Geometry check sheet. Reference: the model listing, model coordinates, mm. A direction names the side the tool comes from. Round coordinates to 2 decimals unless told otherwise and drop trailing zeros. Write each loop counter-clockwise with the first axis right and the second up, starting at its lowest first coordinate (ties: lowest second). Pieces come first, ordered by that corner, then holes. Notation, with made-up numbers: M 40.5,57.5 L 94.5,57.5 A26 ccw 94.5,92.5 Z; hole C 1,-25 d10. An arc over 180 degrees is marked long. Put each result on its own line as item: value. Start each with the question number.
(1) Section check D-D on x = 3.5. Record the cut outline in (y, z), then the cut area to 3 significant figures.
(2) Tool access check on faces 4 (the flat face through (-19.404, -19.269, 5.358)), 5 (the flat face through (9.525, 27, 5)), 6 (the flat face through (2, 31, 2.54)), 7 (the flat face through (0, 0, 2.54)), 8 (the flat face through (8.273, 28.333, 7.862)). Record the directions out of +Z, -Z, +X, -X, +Y, -Y that give a thin tool (end or side, any length) a straight path to the whole face; none if there is none.
(3) Mould release check, pull along Y, two halves, no side actions. Record for faces 1 (the flat face through (-28, -14, 2.54)), 2 (the flat face through (-9.525, 27, 5)), 3 (the flat face through (28.674, -7.002, 7.862)): pulls with the +Y half, pulls with the -Y half, needs draft (parallel to the pull), parting line crosses it, or undercut.
(4) Section check A-A on z = 26. Record the cut outline in (x, y) (1 decimal), then the cut area to 3 significant figures.
(5) Material ranges on probe 1 along X at (y, z) = (25.5, 10) (3 decimals); probe 2 along X at (y, z) = (-6, 11); probe 3 along Y at (x, z) = (0, 1.35), recorded low to high.
(6) Section check B-B on y = 0. Record the cut outline in (x, z) (3 decimals), then the cut area to 3 significant figures.
(7) Gauge pin test, flat ends, axial feed: pin 1 (3 mm diameter, centred on x = -5.5, z = 9, fed in from -Y); pin 2 (1 mm diameter, centred on y = 17.5, z = 18, fed in from -X); pin 3 (5 mm diameter, centred on y = 28, z = 9.5, fed in from +X) (3 decimals). Record the tip position at first contact, or that the pin passes through.
(8) Section check C-C on x = 18. Record the cut outline in (y, z) (3 decimals).
from build123d import *

# Parameters (mm, degrees)
F0_R     = 21.082
F0_R_2   = 2.38125
F1_DEPTH = 2.54
F2_DEPTH = 33.02
F4_DEPTH = 2.54
F6_COUNT = 3
F6_ANGLE = 240


with BuildPart() as f1:
    # F0 (on Top) → F1 (new body)
    with BuildSketch(Plane.XY):
        with BuildLine():
            Line((-9.525, 22.86), (9.525, 22.86))
            ThreePointArc((9.525, 22.86), (0, 24.765), (-9.525, 22.86))
        make_face()
        with BuildLine():
            ThreePointArc((20.6097123392, 13.7311682786), (15.7435419805, 19.1166448654), (9.525, 22.86))
            Line((9.525, 22.86), (-9.525, 22.86))
            ThreePointArc((-9.525, 22.86), (-15.7435419805, 19.1166448654), (-20.6097123392, 13.7311682786))
            ThreePointArc((-20.6097123392, 13.7311682786), (-20.059758407, 13.154112914), (-19.8596191247, 12.3825))
            ThreePointArc((-19.8596191247, 12.3825), (-20.631435956, 11.0205832558), (-22.1963967225, 10.9829503112))
            ThreePointArc((-22.1963967225, 10.9829503112), (-24.4272710788, 4.075984868), (-24.5598407305, -3.181108029))
            Line((-24.5598407305, -3.181108029), (-15.0348407305, -19.678891971))
            ThreePointArc((-15.0348407305, -19.678891971), (-8.6837290983, -23.1926297333), (-1.5866843833, -24.7141185897))
            ThreePointArc((-1.5866843833, -24.7141185897), (0, -23.1775), (1.5866843833, -24.7141185897))
            ThreePointArc((1.5866843833, -24.7141185897), (8.6837290983, -23.1926297333), (15.0348407305, -19.678891971))
            Line((15.0348407305, -19.678891971), (24.5598407305, -3.181108029))
            ThreePointArc((24.5598407305, -3.181108029), (24.7136569602, -1.5938584173), (24.765, 0))
            ThreePointArc((24.765, 0), (24.1143006309, 5.6396569119), (22.1963967225, 10.9829503112))
            ThreePointArc((22.1963967225, 10.9829503112), (20.0723037962, 11.58875), (20.6097123392, 13.7311682786))
        make_face()
        Circle(F0_R, mode=Mode.SUBTRACT)
        with BuildLine():
            ThreePointArc((-9.525, 22.86), (0, 24.765), (9.525, 22.86))
            Line((9.525, 22.86), (9.525, 33.655))
            ThreePointArc((9.525, 33.655), (6.7351920908, 40.3901920908), (0, 43.18))
            ThreePointArc((0, 43.18), (-6.7351920908, 40.3901920908), (-9.525, 33.655))
            Line((-9.525, 33.655), (-9.525, 22.86))
        make_face()
        with Locations((0, 33.655)):
            Circle(F0_R_2, mode=Mode.SUBTRACT)
        with BuildLine():
            ThreePointArc((23.0346191247, 12.3825), (22.2187320387, 13.7698607177), (20.6097123392, 13.7311682786))
            ThreePointArc((20.6097123392, 13.7311682786), (21.4471191247, 12.3825), (22.1963967225, 10.9829503112))
            ThreePointArc((22.1963967225, 10.9829503112), (22.809035869, 11.5668168313), (23.0346191247, 12.3825))
        make_face()
        with BuildLine():
            ThreePointArc((22.1963967225, 10.9829503112), (21.4471191247, 12.3825), (20.6097123392, 13.7311682786))
            ThreePointArc((20.6097123392, 13.7311682786), (20.0723037962, 11.58875), (22.1963967225, 10.9829503112))
        make_face()
        with BuildLine():
            ThreePointArc((-19.8596191247, 12.3825), (-20.059758407, 13.154112914), (-20.6097123392, 13.7311682786))
            ThreePointArc((-20.6097123392, 13.7311682786), (-21.4471191247, 12.3825), (-22.1963967225, 10.9829503112))
            ThreePointArc((-22.1963967225, 10.9829503112), (-20.631435956, 11.0205832558), (-19.8596191247, 12.3825))
        make_face()
        with BuildLine():
            ThreePointArc((-22.1963967225, 10.9829503112), (-21.4471191247, 12.3825), (-20.6097123392, 13.7311682786))
            ThreePointArc((-20.6097123392, 13.7311682786), (-22.8219344532, 13.17625), (-22.1963967225, 10.9829503112))
        make_face()
        with BuildLine():
            Line((-15.0348407305, -19.678891971), (-24.5598407305, -3.181108029))
            ThreePointArc((-24.5598407305, -3.181108029), (-21.4471191247, -12.3825), (-15.0348407305, -19.678891971))
        make_face()
        with BuildLine():
            ThreePointArc((-15.0348407305, -19.678891971), (-21.4471191247, -12.3825), (-24.5598407305, -3.181108029))
            Line((-24.5598407305, -3.181108029), (-33.9085849644, -8.578608029))
            ThreePointArc((-33.9085849644, -8.578608029), (-38.3465284598, -14.3622485954), (-37.3949769354, -21.59))
            ThreePointArc((-37.3949769354, -21.59), (-31.611336369, -26.0279434954), (-24.3835849644, -25.076391971))
            Line((-24.3835849644, -25.076391971), (-15.0348407305, -19.678891971))
        make_face()
        with Locations((-29.1460849644, -16.8275)):
            Circle(F0_R_2, mode=Mode.SUBTRACT)
        with BuildLine():
            Line((33.9085849644, -8.578608029), (24.5598407305, -3.181108029))
            ThreePointArc((24.5598407305, -3.181108029), (21.4471191247, -12.3825), (15.0348407305, -19.678891971))
            Line((15.0348407305, -19.678891971), (24.3835849644, -25.076391971))
            ThreePointArc((24.3835849644, -25.076391971), (31.611336369, -26.0279434954), (37.3949769354, -21.59))
            ThreePointArc((37.3949769354, -21.59), (38.3465284598, -14.3622485954), (33.9085849644, -8.578608029))
        make_face()
        with Locations((29.1460849644, -16.8275)):
            Circle(F0_R_2, mode=Mode.SUBTRACT)
        with BuildLine():
            ThreePointArc((15.0348407305, -19.678891971), (21.4471191247, -12.3825), (24.5598407305, -3.181108029))
            Line((24.5598407305, -3.181108029), (15.0348407305, -19.678891971))
        make_face()
        with BuildLine():
            ThreePointArc((1.5866843833, -24.7141185897), (0, -23.1775), (-1.5866843833, -24.7141185897))
            ThreePointArc((-1.5866843833, -24.7141185897), (0, -24.765), (1.5866843833, -24.7141185897))
        make_face()
        with BuildLine():
            ThreePointArc((1.5866843833, -24.7141185897), (0, -24.765), (-1.5866843833, -24.7141185897))
            ThreePointArc((-1.5866843833, -24.7141185897), (-0.0254439735, -26.3522960827), (1.5875, -24.765))
            ThreePointArc((1.5875, -24.765), (1.5872960827, -24.7395560265), (1.5866843833, -24.7141185897))
        make_face()
        Circle(F0_R)
    extrude(amount=F1_DEPTH)

    # F0 (on Top) → F2 (join)
    with BuildSketch(Plane.XY):
        with BuildLine():
            ThreePointArc((20.6097123392, 13.7311682786), (15.7435419805, 19.1166448654), (9.525, 22.86))
            Line((9.525, 22.86), (-9.525, 22.86))
            ThreePointArc((-9.525, 22.86), (-15.7435419805, 19.1166448654), (-20.6097123392, 13.7311682786))
            ThreePointArc((-20.6097123392, 13.7311682786), (-20.059758407, 13.154112914), (-19.8596191247, 12.3825))
            ThreePointArc((-19.8596191247, 12.3825), (-20.631435956, 11.0205832558), (-22.1963967225, 10.9829503112))
            ThreePointArc((-22.1963967225, 10.9829503112), (-24.4272710788, 4.075984868), (-24.5598407305, -3.181108029))
            Line((-24.5598407305, -3.181108029), (-15.0348407305, -19.678891971))
            ThreePointArc((-15.0348407305, -19.678891971), (-8.6837290983, -23.1926297333), (-1.5866843833, -24.7141185897))
            ThreePointArc((-1.5866843833, -24.7141185897), (0, -23.1775), (1.5866843833, -24.7141185897))
            ThreePointArc((1.5866843833, -24.7141185897), (8.6837290983, -23.1926297333), (15.0348407305, -19.678891971))
            Line((15.0348407305, -19.678891971), (24.5598407305, -3.181108029))
            ThreePointArc((24.5598407305, -3.181108029), (24.7136569602, -1.5938584173), (24.765, 0))
            ThreePointArc((24.765, 0), (24.1143006309, 5.6396569119), (22.1963967225, 10.9829503112))
            ThreePointArc((22.1963967225, 10.9829503112), (20.0723037962, 11.58875), (20.6097123392, 13.7311682786))
        make_face()
        Circle(F0_R, mode=Mode.SUBTRACT)
        with BuildLine():
            Line((-15.0348407305, -19.678891971), (-24.5598407305, -3.181108029))
            ThreePointArc((-24.5598407305, -3.181108029), (-21.4471191247, -12.3825), (-15.0348407305, -19.678891971))
        make_face()
        with BuildLine():
            ThreePointArc((-19.8596191247, 12.3825), (-20.059758407, 13.154112914), (-20.6097123392, 13.7311682786))
            ThreePointArc((-20.6097123392, 13.7311682786), (-21.4471191247, 12.3825), (-22.1963967225, 10.9829503112))
            ThreePointArc((-22.1963967225, 10.9829503112), (-20.631435956, 11.0205832558), (-19.8596191247, 12.3825))
        make_face()
        with BuildLine():
            ThreePointArc((-22.1963967225, 10.9829503112), (-21.4471191247, 12.3825), (-20.6097123392, 13.7311682786))
            ThreePointArc((-20.6097123392, 13.7311682786), (-22.8219344532, 13.17625), (-22.1963967225, 10.9829503112))
        make_face()
        with BuildLine():
            ThreePointArc((22.1963967225, 10.9829503112), (21.4471191247, 12.3825), (20.6097123392, 13.7311682786))
            ThreePointArc((20.6097123392, 13.7311682786), (20.0723037962, 11.58875), (22.1963967225, 10.9829503112))
        make_face()
        with BuildLine():
            ThreePointArc((23.0346191247, 12.3825), (22.2187320387, 13.7698607177), (20.6097123392, 13.7311682786))
            ThreePointArc((20.6097123392, 13.7311682786), (21.4471191247, 12.3825), (22.1963967225, 10.9829503112))
            ThreePointArc((22.1963967225, 10.9829503112), (22.809035869, 11.5668168313), (23.0346191247, 12.3825))
        make_face()
        with BuildLine():
            ThreePointArc((1.5866843833, -24.7141185897), (0, -24.765), (-1.5866843833, -24.7141185897))
            ThreePointArc((-1.5866843833, -24.7141185897), (-0.0254439735, -26.3522960827), (1.5875, -24.765))
            ThreePointArc((1.5875, -24.765), (1.5872960827, -24.7395560265), (1.5866843833, -24.7141185897))
        make_face()
        with BuildLine():
            ThreePointArc((1.5866843833, -24.7141185897), (0, -23.1775), (-1.5866843833, -24.7141185897))
            ThreePointArc((-1.5866843833, -24.7141185897), (0, -24.765), (1.5866843833, -24.7141185897))
        make_face()
        with BuildLine():
            Line((-9.525, 22.86), (9.525, 22.86))
            ThreePointArc((9.525, 22.86), (0, 24.765), (-9.525, 22.86))
        make_face()
        with BuildLine():
            ThreePointArc((15.0348407305, -19.678891971), (21.4471191247, -12.3825), (24.5598407305, -3.181108029))
            Line((24.5598407305, -3.181108029), (15.0348407305, -19.678891971))
        make_face()
    extrude(amount=F2_DEPTH)

    # F3 (on face) → F4 (join)
    with BuildSketch(Plane.YZ.offset(9.525)):
        Polygon((22.86, 13.335), (22.86, 2.54), (33.655, 2.54), align=None)
    extrude(amount=-F4_DEPTH)

    # F5: F1 across plane


with BuildPart() as f1_1:
    add(f1.part)
    add(f1.part.mirror(Plane.YZ))

    # F6: F1 ×3 about axis
    f6_axis = Axis((0, 0, 2.54), (0, 0, -1))


with BuildPart() as f1_2:
    add(f1_1.part)
    for i in range(1, F6_COUNT):
        add(f1_1.part.rotate(f6_axis, i * F6_ANGLE / (F6_COUNT - 1)))


solid = f1_2.part
Answers follow:
1. outline: M -24.52,0 L 42.51,0 L 42.51,2.54 L 24.52,2.54 L 24.52,33.02 L 20.79,33.02 L 20.79,2.54 L -20.79,2.54 L -20.79,33.02 L -24.52,33.02 Z
1. area: 397 mm^2
2. face 4: +Z, -X
2. face 5: +Z, -Z, +X, +Y
2. face 6: +Z, +Y
2. face 7: +Z
2. face 8: +Z, +X, +Y
3. face 1: undercut
3. face 2: needs draft
3. face 3: pulls with the -Y half
4. outline: M -22.2,11 A24.8 ccw -1.6,-24.7 A1.6 ccw long 1.6,-24.7 A24.8 ccw 22.2,11 A1.6 ccw long 20.6,13.7 A24.8 ccw -20.6,13.7 A1.6 ccw long Z; hole C 0,0 d42.2
4. area: 543 mm^2
5. probe 1: x = -9.525 to -6.985, 6.985 to 9.525
5. probe 2: x = -25.63 to -24.36, -24.03 to -20.21, 20.21 to 24.03, 24.36 to 25.63
5. probe 3: y = -26.35 to 31.27, 36.04 to 43.18
6. outline: M -24.765,0 L 24.765,0 L 24.765,33.02 L 21.082,33.02 L 21.082,2.54 L -21.082,2.54 L -21.082,33.02 L -24.765,33.02 Z
6. area: 350 mm^2
7. pin 1: stops at y = -24.44
7. pin 2: stops at x = -18.01
7. pin 3: stops at x = 9.525
8. outline: M -21.391,0 L 17.009,0 L 17.009,33.02 L 10.975,33.02 L 10.975,2.54 L -10.975,2.54 L -10.975,33.02 L -17.009,33.02 L -17.009,2.54 L -18.458,2.54 L -18.458,11.378 L -21.391,9.911 Z
